The model under review builds one solid part; all positions refer to its coordinate system, in mm. A direction names the side the tool comes from. Give positions to 0.01 mm unless a question says otherwise; leave off trailing zeros. Order: outer loops, then holes, each group sorted by start corner. A loop starts at its lowest first (then second) coordinate and runs counter-clockwise, first axis right, second up. Notation, with made-up numbers: (12, -13) - (58, -13) arc R17 ccw to (58, 10) - close; hole circle Ø11 at (65, 64.5). An arc over 180 degrees is marked (long way). Use a Markdown table: item, result. Add a question column.
```python
from build123d import *

# Parameters (mm, degrees)
BOSS_EXTRU_1_DEPTH      = 70
BOSS_EXTRU_2_DEPTH      = 23
ENL_V_MAT_EXTRU_1_REACH = 240.982
ESQUISSE3_R             = 9.500000000000002
COQUE1_T                = -3


with BuildPart() as part:
    # Esquisse1 → Boss.-Extru.1 (new body)
    with BuildSketch(Plane.XY):
        Polygon((0, 0), (-57.85088487178843, 68.94399988070812), (-18.782618272720498, 101.72616797472158), (-3.9985032499301187, 84.10714578298506), (-25.447747657261537, 66.10909271176199), (10.725076137565006, 23.000000000000007), (160, 23.000000000000004), (160, 2.45e-15), align=None)
    extrude(amount=-BOSS_EXTRU_1_DEPTH)

    # Esquisse2 → Boss.-Extru.2 (add)
    with BuildSketch(Plane(origin=(-57.85088487178846, 68.94399988070815, 0), x_dir=(0.7660444431189791, 0.6427876096865383, 0), z_dir=(-0.6427876096865383, 0.7660444431189791, 0))):
        with BuildLine():
            Line((51.00000000000002, 70), (50.99999999999999, 0))
            ThreePointArc((50.99999999999999, 0), (86.00000000000003, 34.999999999999986), (51.00000000000002, 70))
        make_face()
    extrude(amount=-BOSS_EXTRU_2_DEPTH)

    # Esquisse3 → Enlèv. mat.-Extru.1 (cut, up to next)
    with BuildSketch(Plane(origin=(-57.85088487178846, 68.94399988070815, 0), x_dir=(0.7660444431189791, 0.6427876096865383, 0), z_dir=(-0.6427876096865383, 0.7660444431189791, 0)), mode=Mode.PRIVATE) as enl_v_mat_extru_1_sk1:
        with Locations(Location((51.000000000000036, 35, 0), (0, 0, 180))):
            Circle(ESQUISSE3_R)
    enl_v_mat_extru_1_tool1 = extrude(enl_v_mat_extru_1_sk1.sketch, amount=-ENL_V_MAT_EXTRU_1_REACH, mode=Mode.PRIVATE) & part.part
    add(enl_v_mat_extru_1_tool1.solids().sort_by_distance((-18.782618, 101.726168, -35))[0], mode=Mode.SUBTRACT)

    # Coque1
    coque1_openings = [part.faces().sort_by_distance(p)[0] for p in [
        (-27.96387644, 94.022177633, -35),
        (-4.113138552, 99.023139171, -35),
    ]]
    offset(amount=COQUE1_T, openings=coque1_openings, kind=Kind.INTERSECTION)


solid = part.part
```
Q1. We need section B-B (z = -31). Write out the cut boundary in (x, y).
Q2. Machinability: for faces 4 (the flat face through (-7.615, 44.856, -34.51)), 5 (the flat face through (-10.447, 43.565, -34.552)), 6 (the cylindrical face through (12.06, 114.74, -34.3)), which of the approach directions +Z, -Z, +X, -X, +Y, -Y give a long, thin tool a straight path to every point of the face, cutting with its end or side? Answer none if there is none.
Q3. We need section D-D (z = -13). Write out the cut boundary in (x, y).
Q4. Wall thickness on probe 1 along Y at (x, z) = (74.5, -54.5); probe 2 along Z at (x, y) = (-10, 20); probe 3 along Y at (x, z) = (16.5, -30.5): over which ranges is each line inside the solid? List them lowest first.
Q5. Clearance check with flat-ended pins moving along their axes: P1, Ø5, axis at x = 32, z = -62.5, coming from the +Y side; P2, Ø8, axis at y = 54.5, z = -29.5, coming from the +X side; P3, Ø8, axis at x = 3, y = 102.5, coming from the -Z side. State where each tip first meets the part, or that it passes through.
Q6. Draft analysis for pull direction Z (two halves, no side actions). For faces 1 (the flat face through (3.707, 90.573, -35.49)), 2 (the flat face through (-11.244, 81.944, -42.559)), 3 (the cylindrical face through (15.311, 115.532, -34.23)), state which applies: pulls with the +Z half, pulls with the -Z half, needs draft (parallel to the pull), parting line crosses it, or undercut.
Q7. We need section C-C (y = 13). Write out the cut boundary in (x, z), plus the area to 3 significant figures.
Q8. We need section A-A (x = 109.5). Write out the cut boundary in (y, z).
Here are the results:
| question | item | result |
|---|---|---|
| 1 | outline | (-57.85, 68.94) - (0, 0) - (160, 0) - (160, 23) - (10.73, 23) - (-25.45, 66.11) - (-10.6, 78.57) - (-12.53, 80.87) - (-29.67, 66.48) - (9.33, 20) - (157, 20) - (157, 3) - (1.4, 3) - (-55.55, 70.87) - close; (0.67, 91.94) - (2.6, 89.65) - (22.64, 106.46) - (7.85, 124.08) - (5.54, 122.13) - (18.39, 106.81) - close |
| 2 | face 4 | +Z, -Z, +X |
| 2 | face 5 | none |
| 2 | face 6 | -X |
| 3 | outline | (-57.85, 68.94) - (0, 0) - (160, 0) - (160, 23) - (10.73, 23) - (-25.45, 66.11) - (16.85, 101.6) - (2.07, 119.22) - (-0.98, 116.66) - (11.87, 101.34) - (-29.67, 66.48) - (9.33, 20) - (157, 20) - (157, 3) - (1.4, 3) - (-55.55, 70.87) - close |
| 4 | probe 1 | 0 to 3, 20 to 23 |
| 4 | probe 2 | -70 to -67, -3 to 0 |
| 4 | probe 3 | 0 to 3, 20 to 23, 101.31 to 105.22, 108.97 to 113.68 |
| 5 | P1 | y = 23 |
| 5 | P2 | x = -12.35 |
| 5 | P3 | z = -67.42 |
| 6 | face 1 | needs draft |
| 6 | face 2 | undercut |
| 6 | face 3 | parting line crosses it |
| 7 | outline | (-10.91, -70) - (160, -70) - (160, 0) - (-10.91, 0) - close; hole (-6.99, -67) - (157, -67) - (157, -3) - (-6.99, -3) - close |
| 7 | area | 1,470 mm2 |
| 8 | outline | (0, -70) - (23, -70) - (23, 0) - (0, 0) - close; hole (3, -67) - (20, -67) - (20, -3) - (3, -3) - close |
